Work out the finished part from the listing and answer in its coordinate system (mm). A direction names the side the tool comes from. Round coordinates to 2 decimals unless told otherwise and drop trailing zeros. Write each loop counter-clockwise with the first axis right and the second up, starting at its lowest first coordinate (ties: lowest second). Pieces come first, ordered by that corner, then holes.
1. Find section A-A (z = 11). Write down the section's boundary in (x, y).
2. A tool of negligible diameter and unlimited length cuts with its end or side. For faces 1 (the face through (0, 0.3, 0)), 2 (the face through (-8.742, 0.254, -3.992)), from which of +Z, -Z, +X, -X, +Y, -Y can it reach the whole face along a straight path? Write none if from no direction.
3. Find section D-D (x = -5.5). Write down the section's boundary in (y, z).
4. Find section B-B (z = -28.2). Write down the section's boundary in (x, y), and give its area (3 significant figures).
5. Straight lines are drawn through the part: probe 1 along X at (y, z) = (0.3, -28.2); probe 2 along Z at (x, y) = (-5, 0.4) (3 decimals); probe 3 along X at (y, z) = (0.35, -5.5). For each, find the intervals that lie inside material, in ascending order.
6. Find section C-C (y = 0.15). Write down the section's boundary in (x, z), and give its area (3 significant figures).
7. Determine the mould class of faces 3 (the face through (8.177, 0.254, -4.466)), 4 (the face through (0, 0, -8)) for opening direction X: pulls with the +X half, pulls with the -X half, needs draft (parallel to the pull), parting line crosses it, or undercut.
8. Flat-ended cylindrical pins translate along their axes: pin 1 Ø3 at (x, z) = (0, 11) entering from -Y; pin 2 Ø5 at (x, z) = (-1.5, 1) entering from +Y. Find the tip coordinate at first contact, or state that the pin passes through.
Autodesk Inventor part; units mm, degrees
ref_plane "YZ Plane" through (0, 0, 0) normal (1, 0, 0) x (0, 1, 0)
ref_plane "XZ Plane" through (0, 0, 0) normal (0, 1, 0) x (-1, 0, 0)
ref_plane "XY Plane" through (0, 0, 0) normal (0, 0, 1) x (1, 0, 0)
sketch "スケッチ1" plane through (0, 0, 0) normal (0, 1, 0) x (-1, 0, 0)
  line L0 (16, -31) -> (16, 14)
  line L1 (16, 14) -> (-16, 14)
  line L2 (-16, 14) -> (-16, -31)
  line L3 (-16, -31) -> (16, -31)
  line L4 (0, 0) -> (0, -32.6995) construction
  point P0 (0, 14)
  dimension "d0" = 45
  dimension "d1" = 32
  dimension "d2" = 14
extrude "押し出し1" add sketch "スケッチ1" along normal blind 0.5
sketch "スケッチ4" plane through (0, 0.5, 0) normal (0, 1, 0) x (1, 0, 0)
  circle A0 centre (0, -11) radius 1.7
  line L0 (0, 0) -> (-18.7084, 0) construction
  circle A1 centre (-6, 28.2) radius 1.7
  circle A2 centre (6, 28.2) radius 1.7
  line L1 (0, 0) -> (0, 29.6633) construction
  line L2 (16, 31) -> (-16, 31)
  circle A3 centre (9.5263, 5.5) radius 1.7
  circle A4 centre (-9.5263, 5.5) radius 1.7
  point P0 (0, 31)
  dimension "d12" = 3.4
  dimension "d35" = 3.4
  dimension "d36" = 3.4
  dimension "d37" = 6
  dimension "d38" = 2.8
  dimension "d39" = 11
  dimension "d42" = 360
extrude "押し出し3" cut sketch "スケッチ4" against normal through all
sketch "スケッチ6" plane through (0, 0.5, 0) normal (0, 1, 0) x (1, 0, 0)
  circle A0 centre (0, 0) radius 8
  dimension "d44" = 16
extrude "押し出し5" cut sketch "スケッチ6" against normal blind 0.2
properties part number "B_holder_sub_5" material "ステンレス鋼 440C"
Worked answers:
1. outline: (-16, 0) - (-1.7, 0) - (-1.7, 0.5) - (-16, 0.5) - close; (1.7, 0) - (16, 0) - (16, 0.5) - (1.7, 0.5) - close
2. face 1: +Y
2. face 2: +Y, -Y
3. outline: (0, -31) - (0.5, -31) - (0.5, -29.82) - (0, -29.82) - close; (0, -26.58) - (0.5, -26.58) - (0.5, -5.81) - (0.3, -5.81) - (0.3, 5.81) - (0.5, 5.81) - (0.5, 14) - (0, 14) - close
4. outline: (-16, 0) - (-7.7, 0) - (-7.7, 0.5) - (-16, 0.5) - close; (-4.3, 0) - (4.3, 0) - (4.3, 0.5) - (-4.3, 0.5) - close; (7.7, 0) - (16, 0) - (16, 0.5) - (7.7, 0.5) - close
4. area: 12.6 mm2
5. probe 1: x = -16 to -7.7, -4.3 to 4.3, 7.7 to 16
5. probe 2: z = -31 to -29.575, -26.825 to -6.245, 6.245 to 14
5. probe 3: x = -16 to -11.23, -7.83 to -5.81, 5.81 to 7.83, 11.23 to 16
6. outline: (-16, -31) - (16, -31) - (16, 14) - (-16, 14) - close; hole circle Ø3.4 at (-9.53, -5.5); hole circle Ø3.4 at (-6, -28.2); hole circle Ø3.4 at (0, 11); hole circle Ø3.4 at (6, -28.2); hole circle Ø3.4 at (9.53, -5.5)
6. area: 1,390 mm2
7. face 3: undercut
7. face 4: needs draft
8. pin 1: passes through
8. pin 2: stops at y = 0.3
